Source: CAD feature listing. Evaluate the final solid. Frame: model axes, mm. Face numbers are marked on the shaded views. A direction names the side the tool comes from. Give positions to 0.01 mm unless a question says otherwise; leave off trailing zeros. Loops run counter-clockwise (first coordinate to the right, second up) from the corner with the lowest first, then second, coordinate; pieces in that order, holes last. Notation, with made-up numbers: M 51,-4.75 L 109,-4.75 A17 cw 109,18.25 Z; hole C 32,47 d7. An arc over 180 degrees is marked long. Answer in a Markdown table with one row per item.
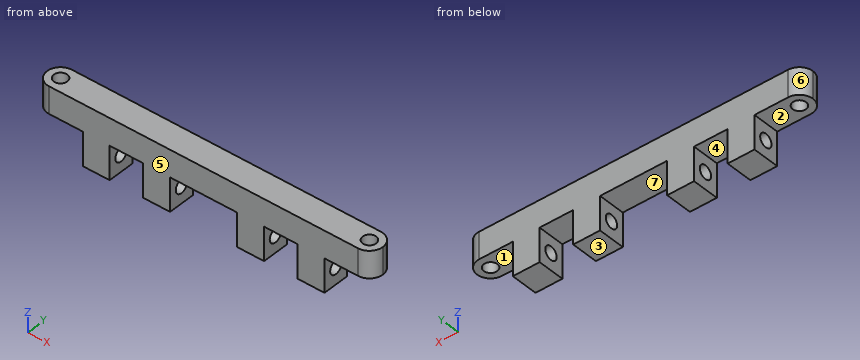
```python
from build123d import *

# Parameters (mm, degrees)
F0_W     = 127
F0_H     = 10.16
F1_DEPTH = 10.16
F2_R     = 5.07999
F3_R     = 2.54
F4_DEPTH = 25.4
F5_W     = 10.16
F5_H     = 10.16
F6_DEPTH = 12.7
F7_R     = 2.54
F8_DEPTH = 99.822


# Not quite as in the source:
# - a fillet or chamfer is up to 0.001 mm smaller than in the source, because OpenCascade refuses the exact size
# - a pattern or mirror of a feature is missing from the dataset's text; its kind, count and spacing are read off the source's solid


with BuildPart() as f1:
    # F0 (on Top) → F1 (new body)
    with BuildSketch(Plane.XY):
        Rectangle(F0_W, F0_H)
    extrude(amount=F1_DEPTH)

    # F2 (radius 5.08 in the source; OpenCascade refuses exactly that, so slightly less here)
    f2_edges = [f1.edges().sort_by_distance(p)[0] for p in [
        (-63.5, -5.08, 5.08),
        (-63.5, 5.08, 5.08),
        (63.5, -5.08, 5.08),
        (63.5, 5.08, 5.08),
    ]]
    fillet(f2_edges, radius=F2_R)

    # F3 (on face) → F4 (cut)
    with BuildSketch(Plane(origin=(0, 0, 0), x_dir=(1, 0, 0), z_dir=(0, 0, -1))):
        with Locations((-58.42, 0)):
            Circle(F3_R)
    f4 = extrude(amount=-F4_DEPTH, mode=Mode.SUBTRACT)

    # F4_copies: F4 across plane
    add(f4.mirror(Plane(origin=(0, 0, 0), x_dir=(0, 0, 1), z_dir=(1, 0, 0))), mode=Mode.SUBTRACT)

    # F5 (on face) → F6 (join)
    with BuildSketch(Plane(origin=(0, 0, 0), x_dir=(1, 0, 0), z_dir=(0, 0, -1))):
        with Locations((-40.64, 0)):
            Rectangle(F5_W, F5_H)
        with Locations((-17.78, 0)):
            Rectangle(F5_W, F5_H)
        with Locations((17.78, 0)):
            Rectangle(F5_W, F5_H)
        with Locations((40.64, 0)):
            Rectangle(F5_W, F5_H)
    extrude(amount=F6_DEPTH)

    # F7 (on face) → F8 (cut)
    with BuildSketch(Plane(origin=(-45.72, 0, 0), x_dir=(0, -1, 0), z_dir=(-1, 0, 0))):
        with Locations((0, -6.35)):
            Circle(F7_R)
    extrude(amount=-F8_DEPTH, mode=Mode.SUBTRACT)


solid = f1.part
```
1) Section A-A, the plane z = -6.35. Count the separate pieces of the cut face and the enclosed holes in it, then the cut area to 3 significant figures.
Reply:
| item | result |
|---|---|
| separate pieces | 8 |
| enclosed holes | 0 |
| area | 206 mm² |
2) Pull-direction query (X, two-part tool) for the marked faces 5, 6 and 7; classes: released by +X, released by -X, zero draft, split by the parting line, or undercut.
Reply:
| item | result |
|---|---|
| face 5 | zero draft |
| face 6 | released by -X |
| face 7 | undercut |
3) Section C-C, the plane x = 17. Return loops of the section in (y, z), then the cut area to 3 significant figures.
Reply:
| item | result |
|---|---|
| outline | M -5.08,-12.7 L 5.08,-12.7 L 5.08,10.16 L -5.08,10.16 Z; hole C 0,-6.35 d5.08 |
| area | 212 mm² |
4) Set-up query: the marked faces 1, 2, 3 and 4. Return all of +Z, -Z, +X, -X, +Y, -Y with unobstructed straight access to the full face (end or side cutting, diameter ignored); none if empty.
Reply:
| item | result |
|---|---|
| face 1 | -Z, +X, +Y, -Y |
| face 2 | -Z, -X, +Y, -Y |
| face 3 | -Z, +X, -X, +Y, -Y |
| face 4 | -Z, +Y, -Y |
5) Pin query (flat end, axial travel): pin 1 Ø3 at (x, y) = (51.5, 1) entering from -Z; pin 2 Ø5 at (y, z) = (-1, -8.5) entering from +X; pin 3 Ø4.5 at (y, z) = (0, -6.35) entering from +X; pin 4 Ø3 at (y, z) = (2, -7.5) entering from -X. Return the tip coordinate at first contact, or that it passes through.
Reply:
| item | result |
|---|---|
| pin 1 | stops at z = 0 |
| pin 2 | stops at x = 45.72 |
| pin 3 | passes through |
| pin 4 | stops at x = -45.72 |
6) Material intervals for L1, parallel to X at y = 0, z = -2; L2, parallel to X at y = 0, z = 7.75; L3, parallel to Z at x = -15, y = 0, sorted ascending.
Reply:
| item | result |
|---|---|
| L1 | x = -45.72 to -35.56, -22.86 to -12.7, 12.7 to 22.86, 35.56 to 45.72 |
| L2 | x = -63.5 to -60.96, -55.88 to 55.88, 60.96 to 63.5 |
| L3 | z = -12.7 to -8.89, -3.81 to 10.16 |
